```python
from build123d import *

# Parameters (mm, degrees)
F1_DEPTH = 3


with BuildPart() as f1:
    # F0 (on Top) → F1 (new body)
    with BuildSketch(Plane.XY):
        with BuildLine():
            Line((75, 15), (-75, 15))
            ThreePointArc((-75, 15), (-78.535534, 13.535534), (-80, 10))
            Line((-80, 10), (-80, -10))
            ThreePointArc((-80, -10), (-78.535534, -13.535534), (-75, -15))
            Line((-75, -15), (-75, -5))
            Line((-75, -5), (-70.25, -5))
            Line((-70.25, -5), (-70.25, -15))
            Line((-70.25, -15), (-2.375, -15))
            Line((-2.375, -15), (-2.375, -5))
            Line((-2.375, -5), (2.375, -5))
            Line((2.375, -5), (2.375, -15))
            Line((2.375, -15), (70.25, -15))
            Line((70.25, -15), (70.25, -5))
            Line((70.25, -5), (75, -5))
            Line((75, -5), (75, -15))
            ThreePointArc((75, -15), (78.535534, -13.535534), (80, -10))
            Line((80, -10), (80, 10))
            ThreePointArc((80, 10), (78.535534, 13.535534), (75, 15))
        make_face()
    extrude(amount=F1_DEPTH)


solid = f1.part
```
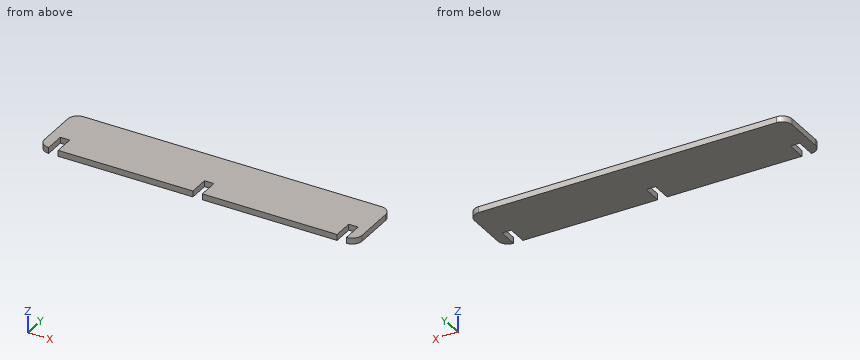
Can you work these out from the model? Positions are in its coordinate system, mm. Round coordinates to 2 decimals unless told otherwise and drop trailing zeros. Loops run counter-clockwise (first coordinate to the right, second up) from the corner with the lowest first, then second, coordinate; pieces in that order, holes last. Notation, with made-up numbers: M 15.25,74.5 L 37.25,74.5 A14 cw 37.25,90.5 Z; hole C 70.5,25 d8. An arc over 180 degrees is marked long. Answer as a JSON object with one key per item and string values. Group by question number.
Q1. Imagine slicing it at B-B, the plane z = 0.5. Please give me the cut outline in (x, y) (3 decimals).
Q2. Please list where these lines run through material, in increasing order: L1, parallel to X at y = -10, z = 1.8 (3 decimals); L2, parallel to X at y = -14, z = 1.3 (3 decimals); L3, parallel to X at y = 11, z = 2.9.
Q3. Imagine slicing it at C-C, the plane y = 13.5. Please give me the cut outline in (x, z), then the cut area to 3 significant figures.
Q4. Imagine slicing it at A-A, the plane y = -13. Please give me the cut outline in (x, z) (3 decimals), then the cut area to 3 significant figures.
Q5. Will these pins go through, and if not, where does the flat tip stop? pin 1 (1.5 mm diameter, centred on y = -11.5, z = 1.5, fed in from -X); pin 2 (1.5 mm diameter, centred on x = -0.5, z = 1, fed in from -Y).
Findings:
{
 "1": {"outline": "M -80,-10 A5 ccw -75,-15 L -75,-5 L -70.25,-5 L -70.25,-15 L -2.375,-15 L -2.375,-5 L 2.375,-5 L 2.375,-15 L 70.25,-15 L 70.25,-5 L 75,-5 L 75,-15 A5 ccw 80,-10 L 80,10 A5 ccw 75,15 L -75,15 A5 ccw -80,10 Z"},
 "2": {"L1": "x = -80 to -75, -70.25 to -2.375, 2.375 to 70.25, 75 to 80", "L2": "x = -78 to -75, -70.25 to -2.375, 2.375 to 70.25, 75 to 78", "L3": "x = -79.9 to 79.9"},
 "3": {"outline": "M -78.57,0 L 78.57,0 L 78.57,3 L -78.57,3 Z", "area": "471 mm2"},
 "4": {"outline": "M -79,0 L -75,0 L -75,3 L -79,3 Z; M -70.25,0 L -2.375,0 L -2.375,3 L -70.25,3 Z; M 2.375,0 L 70.25,0 L 70.25,3 L 2.375,3 Z; M 75,0 L 79,0 L 79,3 L 75,3 Z", "area": "431 mm2"},
 "5": {"pin 1": "stops at x = -79.94", "pin 2": "stops at y = -5"}
}
